Could you check a few things on this model? Use its own coordinates, in mm. Face numbers are marked on the shaded views. A direction names the side the tool comes from. Round coordinates to 2 decimals unless told otherwise and drop trailing zeros. Write each loop counter-clockwise with the first axis right and the second up, starting at its lowest first coordinate (ties: lowest second). Pieces come first, ordered by that corner, then holes. Notation, with made-up numbers: M 87.25,51 L 115.25,51 A19 ccw 115.25,71 Z; hole C 89,-4 d9. An arc over 180 degrees is marked long. One line per item, written item: value. Start each with the question number.
(1) Which directions (+Z, -Z, +X, -X, +Y, -Y) give clear straight access to the entire face, cutting with the end or side of a thin tool? Please do the marked faces 1 and 2.
(2) I want a section at C-C on y = 57.15. Please give me the cut outline in (x, z).
(3) I want a section at D-D on x = 41. Please give me the cut outline in (y, z).
(4) I want a section at A-A on z = 6.5. Please give me the cut outline in (x, y), and give its area (3 significant figures).
(5) I want a section at B-B on x = 0. Please give me the cut outline in (y, z), and give its area (3 significant figures).
(6) If I drill on L1, parallel to X at y = -0.5, z = 4.75; L2, parallel to Y at x = 57.15, z = 3; L3, parallel to Y at x = 0, z = 3.5, over which ranges is the centre line in solid material (lowest first)?
(7) I'm going to push flat-ended pins straight in: pin 1 Ø6 at (x, z) = (-3.5, 5.5) entering from -Y; pin 2 Ø1 at (x, z) = (30.5, 1.5) entering from -Y; pin 3 Ø6 at (y, z) = (52.5, 8) entering from -X. Where does each tip first touch, or does it pass through?
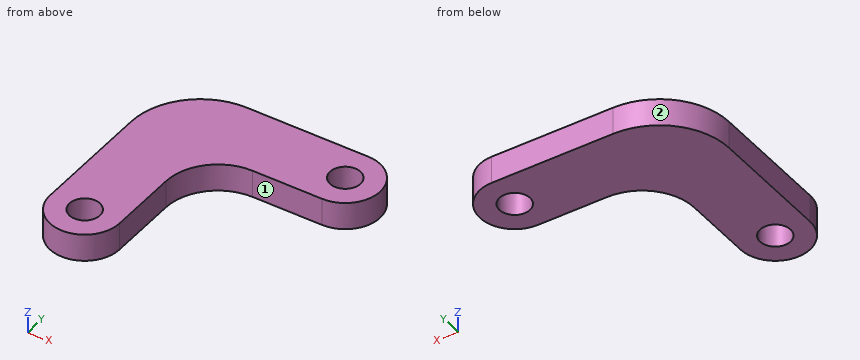
```python
from build123d import *

# Parameters (mm, degrees)
SKETCH1_R           = 5.55625
BOSS_EXTRUDE1_DEPTH = 10


with BuildPart() as part:
    # Sketch1 → Boss-Extrude1 (new body)
    with BuildSketch(Plane.XY):
        with BuildLine():
            ThreePointArc((-12.7, 44.45), (-5.260512242, 62.410512242), (12.7, 69.85))
            Line((12.7, 69.85), (57.15, 69.85))
            ThreePointArc((57.15, 69.85), (69.85, 57.15), (57.15, 44.45))
            Line((57.15, 44.45), (31.75, 44.45))
            ThreePointArc((31.75, 44.45), (18.279615818, 38.870384182), (12.7, 25.4))
            Line((12.7, 25.4), (12.7, 0))
            ThreePointArc((12.7, 0), (0, -12.7), (-12.7, 0))
            Line((-12.7, 0), (-12.7, 44.45))
        make_face()
        with Locations((57.15, 57.15)):
            Circle(SKETCH1_R, mode=Mode.SUBTRACT)
        Circle(SKETCH1_R, mode=Mode.SUBTRACT)
    extrude(amount=BOSS_EXTRUDE1_DEPTH)


solid = part.part
```
Found:
1. face 1: +Z, -Z, +X, -Y
1. face 2: +Z, -Z, -X, +Y
2. outline: M -9.3,0 L 51.59,0 L 51.59,10 L -9.3,10 Z; M 62.71,0 L 69.85,0 L 69.85,10 L 62.71,10 Z
3. outline: M 44.45,0 L 69.85,0 L 69.85,10 L 44.45,10 Z
4. outline: M -12.7,0 A12.7 ccw 12.7,0 L 12.7,25.4 A19.05 cw 31.75,44.45 L 57.15,44.45 A12.7 ccw 57.15,69.85 L 12.7,69.85 A25.4 ccw -12.7,44.45 Z; hole C 0,0 d11.11; hole C 57.15,57.15 d11.11
4. area: 3,160 mm²
5. outline: M -12.7,0 L -5.56,0 L -5.56,10 L -12.7,10 Z; M 5.56,0 L 66.45,0 L 66.45,10 L 5.56,10 Z
5. area: 680 mm²
6. L1: x = -12.69 to -5.53, 5.53 to 12.69
6. L2: y = 44.45 to 51.59, 62.71 to 69.85
6. L3: y = -12.7 to -5.56, 5.56 to 66.45
7. pin 1: stops at y = -12.69
7. pin 2: stops at y = 44.37
7. pin 3: stops at x = -12.19
